from build123d import *

# Parameters (mm, degrees)
SKETCH2_R                              = 16.51
BOSS_EXTRUDE1_DEPTH                    = 398.018
SKETCH3_R                              = 12.7
CUT_EXTRUDE1_DEPTH                     = 398.018
A_0_234_DIAMETER_HOLE1_REACH           = 365.847
A_0_234_DIAMETER_HOLE1_BORE_R          = 2.9718
A_0_234_DIAMETER_HOLE1_ON_FACE_2_REACH = 278.276
A_0_234_DIAMETER_HOLE1_BORE_2_R        = 2.9718
A_0_234_DIAMETER_HOLE1_ON_FACE_3_REACH = 303.949
A_0_234_DIAMETER_HOLE1_BORE_3_R        = 2.9718
N_0_302_DIAMETER_HOLE1_REACH           = 361.923
N_0_302_DIAMETER_HOLE1_BORE_R          = 3.81


with BuildPart() as part:
    # Sketch2 → Boss-Extrude1 (new body)
    with BuildSketch(Plane(origin=(0, 0, 0), x_dir=(1, 0, 0), z_dir=(0, 1, 0))):
        with Locations(Location((0, 0, 0), (0, 0, 270))):
            Circle(SKETCH2_R)
    extrude(amount=BOSS_EXTRUDE1_DEPTH)

    # Sketch3 → Cut-Extrude1 (cut)
    with BuildSketch(Plane.XZ):
        with Locations(Location((0, 0, 0), (0, 0, 270))):
            Circle(SKETCH3_R)
    extrude(amount=-CUT_EXTRUDE1_DEPTH, mode=Mode.SUBTRACT)

    # A (0.234) Diameter Hole1 bore (on position points) → A (0.234) Diameter Hole1 (cut, up to next)
    with BuildSketch(Plane(origin=(-11.22969926, 361.658078854, 12.10264246), x_dir=(0.733049210198, 0, 0.680175606317), z_dir=(-0.680175606317, 0, 0.733049210198)), mode=Mode.PRIVATE) as a_0_234_diameter_hole1_sk1:
        Circle(A_0_234_DIAMETER_HOLE1_BORE_R)
    a_0_234_diameter_hole1_tool1 = extrude(a_0_234_diameter_hole1_sk1.sketch, amount=-A_0_234_DIAMETER_HOLE1_REACH, mode=Mode.PRIVATE) & part.part
    add(a_0_234_diameter_hole1_tool1.solids().sort_by_distance((-11.229699, 361.658079, 12.102642))[0], mode=Mode.SUBTRACT)

    # A (0.234) Diameter Hole1 bore 2 (on position points) → A (0.234) Diameter Hole1 on face 2 (cut, up to next)
    with BuildSketch(Plane(origin=(-10.768707034, 273.389318793, 12.514593434), x_dir=(0.75800069812, 0, 0.652253740234), z_dir=(-0.652253740234, 0, 0.75800069812)), mode=Mode.PRIVATE) as a_0_234_diameter_hole1_on_face_2_sk1:
        Circle(A_0_234_DIAMETER_HOLE1_BORE_2_R)
    a_0_234_diameter_hole1_on_face_2_tool1 = extrude(a_0_234_diameter_hole1_on_face_2_sk1.sketch, amount=-A_0_234_DIAMETER_HOLE1_ON_FACE_2_REACH, mode=Mode.PRIVATE) & part.part
    # A (0.234) Diameter Hole1 bore 2 (on position points) → A (0.234) Diameter Hole1 on face 2 (cut, up to next)
    with BuildSketch(Plane(origin=(-10.768707034, 273.389318793, 12.514593434), x_dir=(0.75800069812, 0, 0.652253740234), z_dir=(-0.652253740234, 0, 0.75800069812)), mode=Mode.PRIVATE) as a_0_234_diameter_hole1_on_face_2_sk2:
        with Locations((0, -91.9723444)):
            Circle(A_0_234_DIAMETER_HOLE1_BORE_2_R)
    a_0_234_diameter_hole1_on_face_2_tool2 = extrude(a_0_234_diameter_hole1_on_face_2_sk2.sketch, amount=-A_0_234_DIAMETER_HOLE1_ON_FACE_2_REACH, mode=Mode.PRIVATE) & part.part
    add(a_0_234_diameter_hole1_on_face_2_tool1.solids().sort_by_distance((-10.768707, 273.389319, 12.514593))[0], mode=Mode.SUBTRACT)
    add(a_0_234_diameter_hole1_on_face_2_tool2.solids().sort_by_distance((-10.768707, 181.416974, 12.514593))[0], mode=Mode.SUBTRACT)

    # A (0.234) Diameter Hole1 bore 3 (on position points) → A (0.234) Diameter Hole1 on face 3 (cut, up to next)
    with BuildSketch(Plane(origin=(-10.291252546, 98.70359084, 12.910082147), x_dir=(0.781955431021, 0, 0.623334343588), z_dir=(-0.623334343588, 0, 0.781955431021)), mode=Mode.PRIVATE) as a_0_234_diameter_hole1_on_face_3_sk1:
        Circle(A_0_234_DIAMETER_HOLE1_BORE_3_R)
    a_0_234_diameter_hole1_on_face_3_tool1 = extrude(a_0_234_diameter_hole1_on_face_3_sk1.sketch, amount=-A_0_234_DIAMETER_HOLE1_ON_FACE_3_REACH, mode=Mode.PRIVATE) & part.part
    add(a_0_234_diameter_hole1_on_face_3_tool1.solids().sort_by_distance((-10.291253, 98.703591, 12.910082))[0], mode=Mode.SUBTRACT)

    # N (0.302) Diameter Hole1 bore (on position points) → N (0.302) Diameter Hole1 (cut, up to next)
    with BuildSketch(Plane(origin=(-5.417804763, 40.200816881, -15.595752356), x_dir=(-0.944624612714, 0, 0.328152923277), z_dir=(-0.328152923277, 0, -0.944624612714)), mode=Mode.PRIVATE) as n_0_302_diameter_hole1_sk1:
        Circle(N_0_302_DIAMETER_HOLE1_BORE_R)
    n_0_302_diameter_hole1_tool1 = extrude(n_0_302_diameter_hole1_sk1.sketch, amount=-N_0_302_DIAMETER_HOLE1_REACH, mode=Mode.PRIVATE) & part.part
    add(n_0_302_diameter_hole1_tool1.solids().sort_by_distance((-5.417805, 40.200817, -15.595752))[0], mode=Mode.SUBTRACT)


solid = part.part
Could you check a few things on this model? Use its own coordinates, in mm. Give positions to 0.01 mm unless a question says otherwise; leave off trailing zeros. Order: outer loops, then holes, each group sorted by start corner. A loop starts at its lowest first (then second) coordinate and runs counter-clockwise, first axis right, second up. Notation, with made-up numbers: (72.25, 16.25) -> (104.25, 16.25) arc R12 ccw to (104.25, 35.25) -> close; hole circle Ø4 at (46, 46.5). An arc over 180 degrees is marked (long way). Answer in a Markdown table with one row per item. Add a question column.
Item 1: Imagine slicing it at B-B (x = 4.5). List the corners of the cut face in (y, z) for me.
Item 2: Imagine slicing it at A-A (z = 0). List the corners of the cut face in (x, y) for me.
Item 3: Please list where these lines run through material, in increasing order: probe 1 along X at (y, z) = (268.5, 0); probe 2 along Z at (x, y) = (4, 84); probe 3 along X at (y, z) = (288, 7.5).
Item 4: I'm going to push flat-ended pins straight in: P1, Ø4, axis at y = 45.5, z = -6, coming from the +X side; P2, Ø5, axis at x = 11.5, y = 133.5, coming from the -Z side; P3, Ø1.5, axis at y = 153.5, z = 10, coming from the -X side. Where does each tip first touch, or does it pass through?
Item 5: We'd pull the mould along Y, two halves only. Please class faces 1 (the flat face through (-9.7, 0, 8.5)), 2 (the cylindrical face through (-10.723, 100.712, 9.938)), 3 (the cylindrical face through (-11.089, 183.425, 9.528)), 4 (the cylindrical face through (-10.05, 196.22, -13.1)): pulls with the +Y half, pulls with the -Y half, needs draft (parallel to the pull), parting line crosses it, or undercut.
Item 6: Imagine slicing it at C-C (y = 337.5). List the corners of the cut face in (x, z) for me.
Result:
| question | item | result |
|---|---|---|
| 1 | outline | (0, -15.88) -> (398.02, -15.88) -> (398.02, -11.88) -> (0, -11.88) -> close; (0, 11.88) -> (398.02, 11.88) -> (398.02, 15.88) -> (0, 15.88) -> close |
| 2 | outline | (-16.51, 0) -> (-12.7, 0) -> (-12.7, 398.02) -> (-16.51, 398.02) -> close; (12.7, 0) -> (16.51, 0) -> (16.51, 398.02) -> (12.7, 398.02) -> close |
| 3 | probe 1 | -16.51 to -12.7, 12.7 to 16.51 |
| 3 | probe 2 | -16.02 to -12.05, 12.05 to 16.02 |
| 3 | probe 3 | -14.71 to -10.25, 10.25 to 14.71 |
| 4 | P1 | x = 16.02 |
| 4 | P2 | z = -13.84 |
| 4 | P3 | x = -13.68 |
| 5 | face 1 | pulls with the -Y half |
| 5 | face 2 | undercut |
| 5 | face 3 | undercut |
| 5 | face 4 | needs draft |
| 6 | outline | circle Ø33.02 at (0, 0); hole circle Ø25.4 at (0, 0) |
